Verification items for the finished model (mm, model axes). A direction names the side the tool comes from. Coordinates: 2 decimals unless noted, no trailing zeros. Write each loop counter-clockwise with the first axis right and the second up, starting at its lowest first coordinate (ties: lowest second). Pieces come first, ordered by that corner, then holes. Notation, with made-up numbers: M 6.5,-34 L 10.5,-34 A10 cw 10.5,-26 Z; hole C 23.5,-38 d1. An arc over 180 degrees is marked long. One line per item, written item: value.
```python
from build123d import *

# Parameters (mm, degrees)
F1_DEPTH = 3


with BuildPart() as f1:
    # F0 (on Right) → F1 (new body)
    with BuildSketch(Plane.YZ):
        with BuildLine():
            ThreePointArc((-25.900381, 34.035096), (-37.900381, 22.035096), (-25.900381, 10.035096))
            Line((-25.900381, 10.035096), (-25.900381, -25.964904))
            Line((-25.900381, -25.964904), (14.099619, -25.964904))
            Line((14.099619, -25.964904), (14.099619, 10.136678))
            ThreePointArc((14.099619, 10.136678), (27.202525, 22.085887), (14.099619, 34.035096))
            Line((14.099619, 34.035096), (-25.900381, 34.035096))
        make_face()
    extrude(amount=F1_DEPTH)


solid = f1.part
```
Item 1: Cross-section at B-B, the plane z = -18. Enter the section's corners in (x, y).
The answers:
outline: M 0,-25.9 L 3,-25.9 L 3,14.1 L 0,14.1 Z
Item 2: Go/stop test with flat-tipped pins: P1, Ø1, axis at x = 1, y = -16, coming from the +Z side; P2, Ø1, axis at x = 0.5, z = -1, coming from the +Y side; P3, Ø1.5, axis at x = 1.5, z = -4, coming from the -Y side. Record where each tip stops, or that it passes through.
The answers:
P1: stops at z = 34.04
P2: stops at y = 14.1
P3: stops at y = -25.9
Item 3: Scan lines: line 1 (Z direction, x = 1.85, y = 7); line 2 (Y direction, x = 0.35, z = 2.5); line 3 (Y direction, x = 1.9, z = 31.5). Record each from-to range of solid material in increasing order.
The answers:
line 1: z = -25.96 to 34.04
line 2: y = -25.9 to 14.1
line 3: y = -33.28 to 22.64
Item 4: Cross-section at A-A, the plane x = 0.6. Enter the section's corners in (y, z).
The answers:
outline: M -25.9,-25.96 L 14.1,-25.96 L 14.1,10.14 A12 ccw long 14.1,34.04 L -25.9,34.04 A12 ccw -25.9,10.04 Z
Item 5: Cross-section at C-C, the plane y = 15.5. Enter the section's corners in (x, z).
The answers:
outline: M 0,10.09 L 3,10.09 L 3,34.08 L 0,34.08 Z
Item 6: Access from +Z, -Z, +X, -X, +Y, -Y to the whole of each face (thin tool, end or side, straight path). Record for faces 1 (the face through (1, -25.9, -8)), 2 (the face through (3, -6, 11)).
The answers:
face 1: -Z, +X, -X, -Y
face 2: +Z, -Z, +X, +Y, -Y
